```python
from build123d import *

# Parameters (mm, degrees)
BOSS_EXTRUDE1_DEPTH  = 20
SKETCH2_W            = 14
SKETCH2_H            = 4
CUT_EXTRUDE1_DEPTH   = 3
SKETCH9_W            = 10.2
SKETCH9_H            = 1
BOSS_EXTRUDE11_DEPTH = 10
SKETCH10_R           = 1.1
CUT_EXTRUDE2_DEPTH   = 5
SKETCH11_R           = 1.1
CUT_EXTRUDE3_DEPTH   = 5


with BuildPart() as part:
    # Sketch1 → Boss-Extrude1 (new body)
    with BuildSketch(Plane.XY):
        Polygon((0, 11), (0, -8), (8.2, -8), (8.2, -18), (10.2, -18), (10.2, -6), (10.2, 11), (8.2, 11), (8.2, 2), (7.2, 2), (7.2, -6), (3, -6), (3, 2), (2, 2), (2, 11), align=None)
    extrude(amount=BOSS_EXTRUDE1_DEPTH)

    # Sketch2 → Cut-Extrude1 (cut)
    with BuildSketch(Plane.ZY):
        with Locations((10, -4)):
            Rectangle(SKETCH2_W, SKETCH2_H)
    extrude(amount=-CUT_EXTRUDE1_DEPTH, mode=Mode.SUBTRACT)

    # Sketch9 → Boss-Extrude11 (add)
    with BuildSketch(Plane(origin=(0, 11, 0), x_dir=(1, 0, 0), z_dir=(0, 1, 0))):
        with Locations((5.1, 0.5)):
            Rectangle(SKETCH9_W, SKETCH9_H)
        with Locations((5.1, -20.5)):
            Rectangle(SKETCH9_W, SKETCH9_H)
    extrude(amount=-BOSS_EXTRUDE11_DEPTH)

    # Sketch10 → Cut-Extrude2 (cut)
    with BuildSketch(Plane.ZY):
        with Locations(Location((4, 6.5, 0), (0, 0, 270))):
            Circle(SKETCH10_R)
        with Locations(Location((16, 6.5, 0), (0, 0, 270))):
            Circle(SKETCH10_R)
    extrude(amount=-CUT_EXTRUDE2_DEPTH, mode=Mode.SUBTRACT)

    # Sketch11 → Cut-Extrude3 (cut)
    with BuildSketch(Plane.ZY.offset(-8.2)):
        with Locations((5, -13)):
            Circle(SKETCH11_R)
        with Locations((15, -13)):
            Circle(SKETCH11_R)
    extrude(amount=-CUT_EXTRUDE3_DEPTH, mode=Mode.SUBTRACT)


solid = part.part
```
Geometry: final body of the model. Coordinates: model frame, mm. A direction names the side the tool comes from. Coordinates: 2 decimals unless noted, no trailing zeros. Write each loop counter-clockwise with the first axis right and the second up, starting at its lowest first coordinate (ties: lowest second). Pieces come first, ordered by that corner, then holes. Notation, with made-up numbers: M 80,-28 L 96,-28 A18 ccw 96,-4 Z; hole C 69,-7.5 d9. An arc over 180 degrees is marked long. Answer as CSV lines item,"result". Start each with the question number.
Q1. Mould query, pull axis X, two halves, no side actions, for faces 6 (the flat face through (8.4, 11, 9.8)), 7 (the flat face through (8.2, -13, 10)), 8 (the flat face through (8, 2, 10)). Classes: released by +X, released by -X, zero draft, split by the parting line, or undercut.
Q2. Cut plane C-C on x = 0.5. Return the cut outline in (y, z).
Q3. Pin query (flat end, axial travel): P1, Ø6, axis at x = 4, z = 9, coming from the -Y side; P2, Ø0.9, axis at x = 1, y = -4, coming from the -Z side; P3, Ø5, axis at y = -14, z = 7.5, coming from the -X side. Return the tip coordinate at first contact, or that it passes through.
Q4. Cut plane D-D on y = -0.75. Return the cut outline in (x, z).
Q5. Line query: line 1 (Z direction, x = 7, y = 8.75); line 2 (Y direction, x = 8.8, z = 5); line 3 (X direction, y = 7.75, z = 15.75). Output: solid intervals per line, ascending. Write a range as from..to.
Q6. Cut plane B-B on z = 10. Return the cut outline in (x, y), then the cut area to 3 significant figures.
Q7. Cut plane A-A on y = -13. Return the cut outline in (x, z).
Q8. Reachability of faces 1 (the flat face through (1, -4, 17)), 2 (the flat face through (6.2, -6.3, 20)), 3 (the flat face through (2, 6, 10)), 4 (the flat face through (4, -8, 10)), 5 (the flat face through (4, -6, 10)) from +Z, -Z, +X, -X, +Y, -Y: full face, straight path, thin tool, end or side. Return the list, or none.
Findings below:
1,face 6,"zero draft"
1,face 7,"released by -X"
1,face 8,"undercut"
2,outline,"M -8,0 L 1,0 L 1,-1 L 11,-1 L 11,21 L 1,21 L 1,20 L -8,20 Z; hole M -6,3 L -2,3 L -2,17 L -6,17 Z; hole C 6.5,4 d2.2; hole C 6.5,16 d2.2"
3,P1,"stops at y = -8"
3,P2,"stops at z = 0"
3,P3,"stops at x = 8.2"
4,outline,"M 0,0 L 3,0 L 3,20 L 0,20 Z; M 7.2,0 L 10.2,0 L 10.2,20 L 7.2,20 Z"
5,line 1,"z = -1..0, 20..21"
5,line 2,"y = -18..-14.1, -11.9..11"
5,line 3,"x = 0..2, 8.2..10.2"
6,outline,"M 0,-8 L 8.2,-8 L 8.2,-18 L 10.2,-18 L 10.2,11 L 8.2,11 L 8.2,2 L 7.2,2 L 7.2,-6 L 0,-6 Z; M 0,-2 L 3,-2 L 3,2 L 2,2 L 2,11 L 0,11 Z"
6,area,"112 mm2"
7,outline,"M 8.2,0 L 10.2,0 L 10.2,3.9 L 8.2,3.9 Z; M 8.2,6.1 L 10.2,6.1 L 10.2,13.9 L 8.2,13.9 Z; M 8.2,16.1 L 10.2,16.1 L 10.2,20 L 8.2,20 Z"
8,face 1,"-X"
8,face 2,"+Z, +X, -X, -Y"
8,face 3,"+Y"
8,face 4,"+Z, -Z, -X, -Y"
8,face 5,"none"
